Geometry check sheet. Reference: the model listing, model coordinates, mm. Face numbers are marked on the shaded views. A direction names the side the tool comes from. Coordinates: 2 decimals unless noted, no trailing zeros. Write each loop counter-clockwise with the first axis right and the second up, starting at its lowest first coordinate (ties: lowest second). Pieces come first, ordered by that corner, then holes. Notation, with made-up numbers: M 42,70.5 L 60,70.5 A12 cw 60,93.5 Z; hole C -11.75,71 d6. An arc over 180 degrees is marked long. Put each result on its own line as item: value. Start each with the question number.
1) Scan lines: line 1 along Y through (x, z) = (-12.5, 9) (3 decimals); line 2 along X through (y, z) = (-60, -0.5); line 3 along Z through (x, y) = (-1.5, -60.5). Record each from-to range of solid material in increasing order.
2) Cross-section at B-B on z = 0. Record the cut outline in (x, y) (3 decimals).
3) Cross-section at C-C on y = -9. Record the cut outline in (x, z), plus the area to 3 significant figures.
4) Set-up check for the marked faces 1 and 2: record each of +Z, -Z, +X, -X, +Y, -Y from which the full face is reachable in a straight line by a thin tool's end or side.
5) Gauge pin test, flat ends, axial feed: pin 1 (3 mm diameter, centred on y = -15, z = 8, fed in from +X); pin 2 (10 mm diameter, centred on y = -46.5, z = 9.5, fed in from -X); pin 3 (1.5 mm diameter, centred on x = 9.5, z = 0.5, fed in from -Y) (3 decimals). Record the tip position at first contact, or that the pin passes through.
6) Cross-section at A-A on x = 0. Record the cut outline in (y, z) (3 decimals).
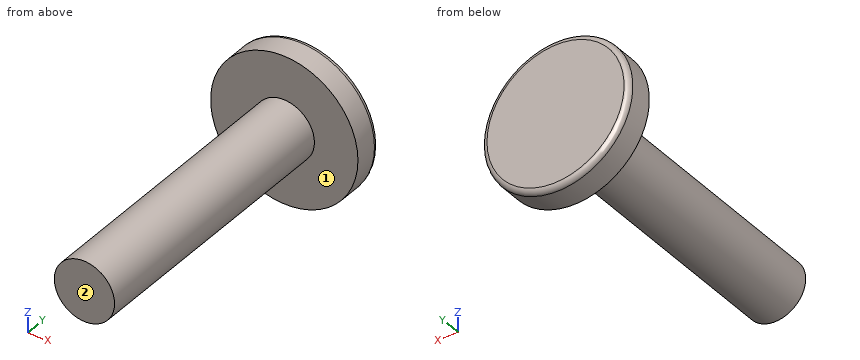
from build123d import *

# Parameters (mm, degrees)
F0_R     = 7.47149
F1_DEPTH = 76.2
F2_R     = 18.271136
F3_DEPTH = 6.985
F4_R     = 1.27


with BuildPart() as f1:
    # F0 (on Front) → F1 (new body)
    with BuildSketch(Plane.XZ):
        Circle(F0_R)
    extrude(amount=F1_DEPTH)

    # F2 (on Front) → F3 (join)
    with BuildSketch(Plane.XZ):
        Circle(F2_R)
    extrude(amount=F3_DEPTH)

    # F4
    f4_edges = [f1.edges().sort_by_distance(p)[0] for p in [
        (-18.271136, 0, 0),
    ]]
    fillet(f4_edges, radius=F4_R)


solid = f1.part
Answer key:
1. line 1: y = -6.985 to 0
1. line 2: x = -7.45 to 7.45
1. line 3: z = -7.32 to 7.32
2. outline: M -18.271,-6.985 L -7.471,-6.985 L -7.471,-76.2 L 7.471,-76.2 L 7.471,-6.985 L 18.271,-6.985 L 18.271,-1.27 A1.27 ccw 17.001,0 L -17.001,0 A1.27 ccw -18.271,-1.27 Z
3. outline: C 0,0 d14.94
3. area: 175 mm²
4. face 1: -Y
4. face 2: +Z, -Z, +X, -X, -Y
5. pin 1: stops at x = 3.68
5. pin 2: stops at x = -5.96
5. pin 3: stops at y = -6.985
6. outline: M -76.2,-7.471 L -6.985,-7.471 L -6.985,-18.271 L -1.27,-18.271 A1.27 ccw 0,-17.001 L 0,17.001 A1.27 ccw -1.27,18.271 L -6.985,18.271 L -6.985,7.471 L -76.2,7.471 Z
